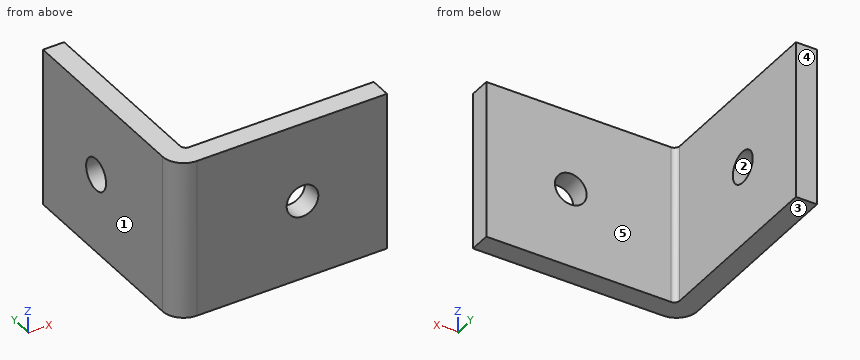
from build123d import *

# Parameters (mm, degrees)
BOSS_EXTRUDE1_DEPTH = 15
SKETCH3_R           = 1.5
CUT_EXTRUDE2_DEPTH  = 3
SKETCH4_R           = 1.5
CUT_EXTRUDE3_DEPTH  = 3


with BuildPart() as part:
    # Sketch1 → Boss-Extrude1 (new body)
    with BuildSketch(Plane.XY):
        with BuildLine():
            Line((0, 2), (0, 20))
            Line((0, 20), (2, 20))
            Line((2, 20), (2, 2.5))
            ThreePointArc((2, 2.5), (2.146446609, 2.146446609), (2.5, 2))
            Line((2.5, 2), (20, 2))
            Line((20, 2), (20, 0))
            Line((20, 0), (2, 0))
            ThreePointArc((2, 0), (0.585786438, 0.585786438), (0, 2))
        make_face()
    extrude(amount=BOSS_EXTRUDE1_DEPTH)

    # Sketch3 → Cut-Extrude2 (cut, through all)
    with BuildSketch(Plane(origin=(0, 2, 0), x_dir=(1, 0, 0), z_dir=(0, 1, 0))):
        with Locations((12, -7.5)):
            Circle(SKETCH3_R)
    extrude(amount=-CUT_EXTRUDE2_DEPTH, mode=Mode.SUBTRACT)

    # Sketch4 → Cut-Extrude3 (cut, through all)
    with BuildSketch(Plane(origin=(2, 0, 0), x_dir=(0, 0, -1), z_dir=(1, 0, 0))):
        with Locations((-7.5, 12)):
            Circle(SKETCH4_R)
    extrude(amount=-CUT_EXTRUDE3_DEPTH, mode=Mode.SUBTRACT)


solid = part.part
The model under review builds one solid part; all positions refer to its coordinate system, in mm. Face numbers are marked on the shaded views. A direction names the side the tool comes from. Give positions to 0.01 mm unless a question says otherwise; leave off trailing zeros. Loops run counter-clockwise (first coordinate to the right, second up) from the corner with the lowest first, then second, coordinate; pieces in that order, holes last. Notation, with made-up numbers: (44, 69.25) -> (69, 69.25) arc R24 ccw to (69, 97.25) -> close; hole circle Ø10 at (16.25, 63.25). An arc over 180 degrees is marked (long way). Answer as a JSON object with one key per item and string values. Group by question number.
Q1. Insertion check: pin 1 (4 mm diameter, centred on x = 16, z = 5, fed in from +Y); pin 2 (8 mm diameter, centred on y = 16.5, z = 5.5, fed in from -X); pin 3 (7.5 mm diameter, centred on y = 9, z = 10, fed in from +X). Each pin has a flat end and moves straight along its axis. Give the tip position at first contact, or say it passes through.
Q2. Take a section at A-A (x = 12). Write out the cut boundary in (y, z), plus the area to 3 significant figures.
Q3. Wall thickness on line 1 along X through (y, z) = (16, 5.75); line 2 along Y through (x, z) = (0.8, 7.5): over which ranges is each line inside the solid? List them lowest first.
Q4. Take a section at C-C (z = 7.5). Write out the cut boundary in (x, y).
Q5. Take a section at D-D (z = 14.25). Write out the cut boundary in (x, y).
Q6. Tool access review of the marked faces 4 and 5: name each direction out of +Z, -Z, +X, -X, +Y, -Y from which nothing blocks a thin tool from reaching the whole face with its end or side.
Q7. Draft analysis for pull direction Z (two halves, no side actions). For the marked faces 1, 2 and 3, state which applies: pulls with the +Z half, pulls with the -Z half, needs draft (parallel to the pull), parting line crosses it, or undercut.
Answer below:
{
 "1": {"pin 1": "stops at y = 2", "pin 2": "stops at x = 0", "pin 3": "stops at x = 2"},
 "2": {"outline": "(0, 0) -> (2, 0) -> (2, 6) -> (0, 6) -> close; (0, 9) -> (2, 9) -> (2, 15) -> (0, 15) -> close", "area": "24.0 mm2"},
 "3": {"line 1": "x = 0 to 2", "line 2": "y = 0.4 to 10.5, 13.5 to 20"},
 "4": {"outline": "(0, 2) arc R2 ccw to (2, 0) -> (10.5, 0) -> (10.5, 2) -> (2.5, 2) arc R0.5 cw to (2, 2.5) -> (2, 10.5) -> (0, 10.5) -> close; (0, 13.5) -> (2, 13.5) -> (2, 20) -> (0, 20) -> close; (13.5, 0) -> (20, 0) -> (20, 2) -> (13.5, 2) -> close"},
 "5": {"outline": "(0, 2) arc R2 ccw to (2, 0) -> (20, 0) -> (20, 2) -> (2.5, 2) arc R0.5 cw to (2, 2.5) -> (2, 20) -> (0, 20) -> close"},
 "6": {"face 4": "+Z, -Z, +X, -X, +Y", "face 5": "+Z, -Z, +X, +Y"},
 "7": {"face 1": "needs draft", "face 2": "undercut", "face 3": "pulls with the -Z half"}
}
